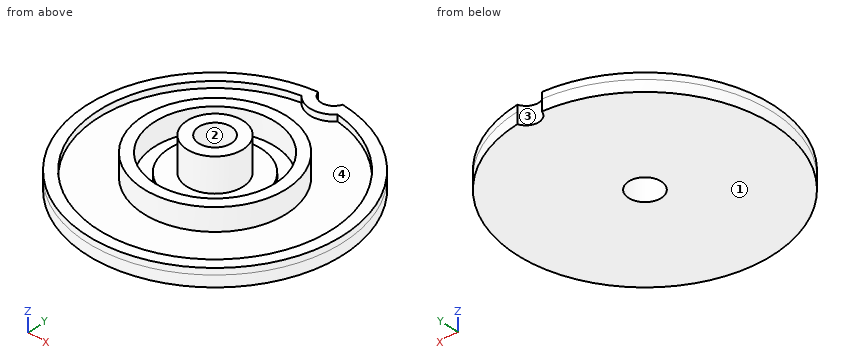
Autodesk Inventor part; units mm, degrees
ref_plane "Work Plane1" through (0, 0, 1) normal (0, 0, 1) x (1, 0, 0)
ref_plane "Work Plane2" through (0, 0, 1) normal (0, 0, 1) x (1, 0, 0)
ref_plane "YZ Plane" through (0, 0, 0) normal (1, 0, 0) x (0, 1, 0)
sketch "Sketch1" plane through (0, 0, 0) normal (0, 0, 1) x (1, 0, 0)
  circle A0 centre (0, 0) radius 11.4
  dimension "d0" = 22.8
extrude "Extrusion1" add sketch "Sketch1" along normal blind 1
ref_plane "Work Plane1" through (0, 0, 1) normal (0, 0, 1) x (1, 0, 0)
sketch "Sketch3" plane through (0, 0, 1) normal (0, 0, 1) x (1, 0, 0)
  circle A0 centre (0, 0) radius 6.375
  circle A1 centre (0, 0) radius 5.375
  dimension "d6" = 12.75
  dimension "d7" = 10.75
extrude "Extrusion3" add sketch "Sketch3" along normal blind 2
ref_plane "Work Plane2" through (0, 0, 1) normal (0, 0, 1) x (1, 0, 0)
sketch "Sketch5" plane through (0, 0, 1) normal (0, 0, 1) x (1, 0, 0)
  circle A0 centre (0, 0) radius 4.125
  dimension "d14" = 8.25
extrude "Extrusion5" add sketch "Sketch5" along normal blind 0.4
sketch "Sketch6" plane through (0, 0, 0) normal (0, 0, -1) x (-1, 0, 0)
  circle A0 centre (0, 0) radius 1.45
  dimension "d17" = 2.9
extrude "Extrusion6" cut sketch "Sketch6" against normal up to surface (1.4 mm away)
sketch "Sketch7" plane through (0, 0, 1.4) normal (0, 0, 1) x (1, 0, 0)
  circle A0 centre (0, 0) radius 1.45
  circle A1 centre (0, 0) radius 1.45
  circle A2 centre (0, 0) radius 2.5
  dimension "d20" = 5
extrude "Pressguide" add sketch "Sketch7" along normal blind 3
sketch "Sketch8" plane through (0, 0, 1) normal (0, 0, 1) x (1, 0, 0)
  circle A0 centre (0, 0) radius 11.4
  line L0 (-1.1, 11.3468) -> (1.1, 11.3468) construction
  line L1 (0, 11.3468) -> (0, 10.5468) construction
  arc A1 (-1.1, 11.3468) -> (1.1, 11.3468) centre (0, 11.7031) ccw
  dimension "d23" = 2.2
  dimension "d24" = 0.8
extrude "Extrusion8" cut sketch "Sketch8" against normal up to surface (1 mm away) contours A1 A0 picked at (-0.044, 11.1142)
sketch "Sketch9" plane through (0, 0, 1) normal (0, 0, 1) x (1, 0, 0)
  arc A0 (-1.1, 11.3468) -> (1.1, 11.3468) centre (0, 0) ccw
  arc A1 (-1.1, 11.3468) -> (1.1, 11.3468) centre (0, 11.7031) ccw
  arc A2 (-1.6146, 10.2739) -> (1.6146, 10.2739) centre (0, 0) ccw
  arc A3 (-1.6146, 10.2739) -> (1.6146, 10.2739) centre (0, 11.7031) ccw
  dimension "d27" = 1
extrude "Extrusion9" add sketch "Sketch9" along normal blind 0.57
sketch "Sketch10" plane through (0, 0, 0) normal (0, 0, -1) x (-1, 0, 0)
  circle A0 centre (0, 0) radius 1.45
extrude "Axle" [suppressed]
properties part number "PMSealNoAxle"
Here's how the part is built. I have some questions about the finished solid (model axes, mm). Face numbers are marked on the shaded views. A direction names the side the tool comes from. Round coordinates to 2 decimals unless told otherwise and drop trailing zeros. Loops run counter-clockwise (first coordinate to the right, second up) from the corner with the lowest first, then second, coordinate; pieces in that order, holes last. Notation, with made-up numbers: M 71,85.5 L 79,85.5 A17 ccw 79,93.5 Z; hole C 34,-5 d3. An arc over 180 degrees is marked long. Write each question's results on one line, items separated by ' | '. Start each with the question number.
(1) I want a section at B-B (y = 0). Please give me the cut outline in (x, z) (3 decimals), then the cut area to 3 significant figures.
(2) On a 3-axis mill with a long thin cutter (end or side, diameter ignored), from which of +Z, -Z, +X, -X, +Y, -Y can I reach the whole of each face in a straight line? I mean the marked faces 3 and 4. Say none if no direction works.
(3) Will these pins go through, and if not, where does the flat tip stop? P1, Ø1, axis at x = -5.5, y = 3, coming from the +Z side; P2, Ø6.5, axis at x = 2, y = 2, coming from the +Z side; P3, Ø1.5, axis at x = -7, y = -2.5, coming from the +Z side; P4, Ø6, axis at x = -9, y = 4, coming from the +Z side.
(4) If I drill on probe 1 along Y at (x, z) = (0, 1.6) (3 decimals); probe 2 along Z at (x, y) = (-3, 7.25); probe 3 along X at (y, z) = (-2, 1.85), over which ranges is the centre line in solid material (lowest first)? Write a range as from..to.
(5) Thinking about a two-plate mould opening in X: for the marked faces 1 and 2, which applies, pulls with the +X half, pulls with the -X half, needs draft (parallel to the pull), parting line crosses it, or undercut?
(6) I want a section at D-D (x = -3.75). Please give me the cut outline in (y, z), then the cut area to 3 significant figures.
(7) I want a section at A-A (x = 0). Please give me the cut outline in (y, z) (3 decimals), then the cut area to 3 significant figures.
(8) I want a section at C-C (z = 2.1). Please give me the cut outline in (x, y) (3 decimals), then the cut area to 3 significant figures.
Solved:
1) outline: M -11.4,0 L -1.45,0 L -1.45,4.4 L -2.5,4.4 L -2.5,1.4 L -4.125,1.4 L -4.125,1 L -5.375,1 L -5.375,3 L -6.375,3 L -6.375,1 L -10.4,1 L -10.4,1.57 L -11.4,1.57 Z; M 1.45,0 L 11.4,0 L 11.4,1.57 L 10.4,1.57 L 10.4,1 L 6.375,1 L 6.375,3 L 5.375,3 L 5.375,1 L 4.125,1 L 4.125,1.4 L 2.5,1.4 L 2.5,4.4 L 1.45,4.4 Z | area: 33.5 mm²
2) face 3: +Z, -Z, +Y | face 4: +Z
3) P1: stops at z = 3 | P2: stops at z = 4.4 | P3: stops at z = 1 | P4: stops at z = 1.57
4) probe 1: y = -6.375..-5.375, -2.5..-1.45, 1.45..2.5, 5.375..6.375 | probe 2: z = 0..1 | probe 3: x = -6.05..-4.99, -1.5..1.5, 4.99..6.05
5) face 1: needs draft | face 2: undercut
6) outline: M -10.77,0 L 10.77,0 L 10.77,1.57 L 9.7,1.57 L 9.7,1 L 5.16,1 L 5.16,3 L 3.85,3 L 3.85,1 L 1.72,1 L 1.72,1.4 L -1.72,1.4 L -1.72,1 L -3.85,1 L -3.85,3 L -5.16,3 L -5.16,1 L -9.7,1 L -9.7,1.57 L -10.77,1.57 Z | area: 29.3 mm²
7) outline: M -11.4,0 L -1.45,0 L -1.45,4.4 L -2.5,4.4 L -2.5,1.4 L -4.125,1.4 L -4.125,1 L -5.375,1 L -5.375,3 L -6.375,3 L -6.375,1 L -10.4,1 L -10.4,1.57 L -11.4,1.57 Z; M 1.45,0 L 10.547,0 L 10.547,1.57 L 9.547,1.57 L 9.547,1 L 6.375,1 L 6.375,3 L 5.375,3 L 5.375,1 L 4.125,1 L 4.125,1.4 L 2.5,1.4 L 2.5,4.4 L 1.45,4.4 Z | area: 32.6 mm²
8) outline: C 0,0 d12.75; C 0,0 d5; hole C 0,0 d10.75; hole C 0,0 d2.9 | area: 49.9 mm²
